Source: CAD feature listing. Evaluate the final solid. Frame: model axes, mm. Face numbers are marked on the shaded views. Round coordinates to 2 decimals unless told otherwise and drop trailing zeros. Loops run counter-clockwise (first coordinate to the right, second up) from the corner with the lowest first, then second, coordinate; pieces in that order, holes last.
(1) Material intervals for probe 1 along Y at (x, z) = (-6.25, 0); probe 2 along X at (y, z) = (13, 0); probe 3 along X at (y, z) = (10.75, 3), sorted ascending.
(2) Section D-D, the plane x = -7.5. Return the cut outline in (y, z), plus the area to 3 significant figures.
(3) Section B-B, the plane y = 10.5. Return the cut outline in (x, z), plus the area to 3 significant figures.
(4) Section C-C, the plane z = -4.5. Return the cut outline in (x, y).
(5) Section A-A, the plane x = 0. Return the cut outline in (y, z).
(6) Mould query, pull axis X, two halves, no side actions, for the marked faces 1, 2, 3 and 4. Classes: pulls with the +X half, pulls with the -X half, needs draft (parallel to the pull), parting line crosses it, or undercut.
(7) First-contact query: pin 1 Ø2.5 at (y, z) = (5, 0) entering from -X; pin 2 Ø1.5 at (y, z) = (16, -7) entering from +X; pin 3 Ø5 at (x, z) = (1, -0.5) entering from +Y; pin 4 Ø5 at (y, z) = (9.5, -4.5) entering from -X. Flat tips, straight axial feed; report the tip coordinate or a pass-through.
```python
from build123d import *

# Parameters (mm, degrees)
SKETCH1_R           = 10
SKETCH1_R_2         = 4
BOSS_EXTRUDE1_DEPTH = 20
SKETCH2_R           = 5
CUT_EXTRUDE1_DEPTH  = 10
SKETCH3_R           = 1.65
CUT_EXTRUDE2_DEPTH  = 10


with BuildPart() as part:
    # Sketch1 → Boss-Extrude1 (new body)
    with BuildSketch(Plane(origin=(0, 0, 0), x_dir=(1, 0, 0), z_dir=(0, 1, 0))):
        with Locations(Location((0, 0, 0), (0, 0, 270))):
            Circle(SKETCH1_R)
        with Locations(Location((0, 0, 0), (0, 0, 270))):
            Circle(SKETCH1_R_2, mode=Mode.SUBTRACT)
    extrude(amount=BOSS_EXTRUDE1_DEPTH)

    # Sketch2 → Cut-Extrude1 (cut)
    with BuildSketch(Plane(origin=(0, 20, 0), x_dir=(1, 0, 0), z_dir=(0, 1, 0))):
        with Locations(Location((0, 0, 0), (0, 0, 270))):
            Circle(SKETCH2_R)
    extrude(amount=-CUT_EXTRUDE1_DEPTH, mode=Mode.SUBTRACT)

    # Sketch3 → Cut-Extrude2 (cut)
    with BuildSketch(Plane(origin=(0, 0, 0), x_dir=(0, 0, -1), z_dir=(1, 0, 0))):
        with Locations((0, 5)):
            Circle(SKETCH3_R)
        with Locations((0, 15)):
            Circle(SKETCH3_R)
    extrude(amount=-CUT_EXTRUDE2_DEPTH, mode=Mode.SUBTRACT)


solid = part.part
```
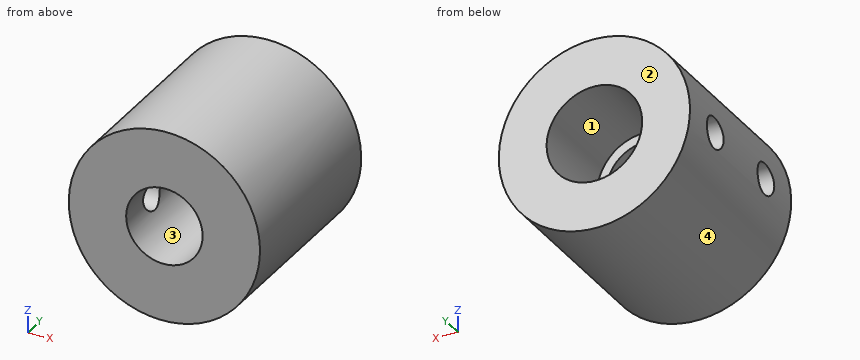
Output values:
1. probe 1: y = 0 to 3.35, 6.65 to 13.35, 16.65 to 20
1. probe 2: x = -10 to -5, 5 to 10
1. probe 3: x = -9.54 to -4, 4 to 9.54
2. outline: (0, -6.61) - (20, -6.61) - (20, 6.61) - (0, 6.61) - close; hole circle Ø3.3 at (5, 0); hole circle Ø3.3 at (15, 0)
2. area: 247 mm2
3. outline: circle Ø20 at (0, 0); hole circle Ø10 at (0, 0)
3. area: 236 mm2
4. outline: (-8.93, 0) - (8.93, 0) - (8.93, 20) - (2.18, 20) - (2.18, 10) - (-2.18, 10) - (-2.18, 20) - (-8.93, 20) - close
5. outline: (0, -10) - (20, -10) - (20, -5) - (10, -5) - (10, -4) - (0, -4) - close; (0, 4) - (10, 4) - (10, 5) - (20, 5) - (20, 10) - (0, 10) - close
6. face 1: undercut
6. face 2: needs draft
6. face 3: undercut
6. face 4: parting line crosses it
7. pin 1: stops at x = 3.8
7. pin 2: stops at x = 7.81
7. pin 3: passes through
7. pin 4: stops at x = -9.8
